CAD build for the part. Positions are in the model's coordinates, mm. A direction names the side the tool comes from. Give positions to 0.01 mm unless a question says otherwise; leave off trailing zeros. Write each loop counter-clockwise with the first axis right and the second up, starting at its lowest first coordinate (ties: lowest second). Pieces come first, ordered by that corner, then holes. Notation, with made-up numbers: (-7.5, 39) -> (3.5, 39) arc R22 cw to (3.5, 58) -> close; hole circle Ø7 at (22, 64.25). An arc over 180 degrees is marked (long way). Answer as a JSON object with one key per item and string values.
```python
from build123d import *

# Parameters (mm, degrees)
F1_DEPTH = 4.5
F2_W     = 0.5
F2_H     = 4.5
F3_DEPTH = 6


with BuildPart() as f1:
    # F0 (on Top) → F1 (new body)
    with BuildSketch(Plane.XY):
        Polygon((-0.469149, 31.306926), (-0.969149, 31.306926), (-0.969149, 8.820471), (-2.198889, 5.306926), (-2.198889, -1.893074), (-0.969149, -5.406618), (-0.969149, -16.696654), (-0.469149, -16.696654), (-0.469149, -5.406618), (0.760592, -1.893074), (0.760592, 5.306926), (-0.469149, 8.820471), align=None)
        Polygon((-1.669149, -1.893074), (-1.669149, 5.306926), (-0.969149, 7.306926), (-0.719149, 8.021212), (-0.469149, 7.306926), (0.230851, 5.306926), (0.230851, -1.893074), (-0.469149, -3.893074), (-0.719149, -4.607359), (-0.969149, -3.893074), align=None, mode=Mode.SUBTRACT)
    extrude(amount=F1_DEPTH)

    # F2 (on face) → F3 (join)
    with BuildSketch(Plane.XY.offset(4.5)):
        with Locations((-0.719149, 29.056926)):
            Rectangle(F2_W, F2_H)
    extrude(amount=F3_DEPTH)


solid = f1.part
```
1) Slice it at C-C (z = 9.25). List the corners of the cut face in (x, y).
Model answer:
{"outline": "(-0.97, 26.81) -> (-0.47, 26.81) -> (-0.47, 31.31) -> (-0.97, 31.31) -> close"}
2) Slice it at B-B (y = -2.5). List the corners of the cut face in (x, z).
Model answer:
{"outline": "(-1.99, 0) -> (-1.46, 0) -> (-1.46, 4.5) -> (-1.99, 4.5) -> close; (0.02, 0) -> (0.55, 0) -> (0.55, 4.5) -> (0.02, 4.5) -> close"}
3) Slice it at D-D (y = 18). List the corners of the cut face in (x, z), then the cut area to 3 significant figures.
Model answer:
{"outline": "(-0.97, 0) -> (-0.47, 0) -> (-0.47, 4.5) -> (-0.97, 4.5) -> close", "area": "2.25 mm2"}
4) Pin check, flat tips, straight feed: pin 1 (5 mm diameter, centred on y = -9.5, z = 2, fed in from +X); pin 2 (0.9 mm diameter, centred on x = -0.5, y = -3.5, fed in from +Z); pin 3 (5 mm diameter, centred on y = -11, z = 2.5, fed in from -X). Stop position of each tip, or through.
Model answer:
{"pin 1": "stops at x = -0.47", "pin 2": "stops at z = 4.5", "pin 3": "stops at x = -0.97"}
5) Slice it at A-A (z = 1.5). List the corners of the cut face in (x, y).
Model answer:
{"outline": "(-2.2, -1.89) -> (-0.97, -5.41) -> (-0.97, -16.7) -> (-0.47, -16.7) -> (-0.47, -5.41) -> (0.76, -1.89) -> (0.76, 5.31) -> (-0.47, 8.82) -> (-0.47, 31.31) -> (-0.97, 31.31) -> (-0.97, 8.82) -> (-2.2, 5.31) -> close; hole (-1.67, -1.89) -> (-0.97, -3.89) -> (-0.72, -4.61) -> (-0.47, -3.89) -> (0.23, -1.89) -> (0.23, 5.31) -> (-0.47, 7.31) -> (-0.72, 8.02) -> (-0.97, 7.31) -> (-1.67, 5.31) -> close"}
6) 3-axis set-ups, long thin cutter, end or side, ignore diameter. For faces 1 (the flat face through (-0.969, 22, 3)), 2 (the flat face through (-2, 4, 4.5)), 3 (the flat face through (-0.469, 22, 3)), 4 (the flat face through (-0.969, -11, 2)): which of +Z, -Z, +X, -X, +Y, -Y reach the whole face in a straight line?
Model answer:
{"face 1": "+Z, -Z, -X, +Y", "face 2": "+Z, +X, -X, -Y", "face 3": "+Z, -Z, +X, +Y", "face 4": "+Z, -Z, -X, -Y"}
7) Wall check: probe 1 along X at (y, z) = (0, 1.5); probe 2 along X at (y, z) = (20, 1.75); probe 3 along Y at (x, z) = (-0.85, 6). Give the ranges that are in metal, low to high.
Model answer:
{"probe 1": "x = -2.2 to -1.67, 0.23 to 0.76", "probe 2": "x = -0.97 to -0.47", "probe 3": "y = 26.81 to 31.31"}
